For this review, use the dimensioned drawing (mm, ordinates from the lowest corner) and the shaded views. Coordinates: 2 decimals unless noted, no trailing zeros. Write each loop counter-clockwise with the first axis right and the second up, starting at its lowest first coordinate (ties: lowest second). Pieces come first, ordered by that corner, then holes.
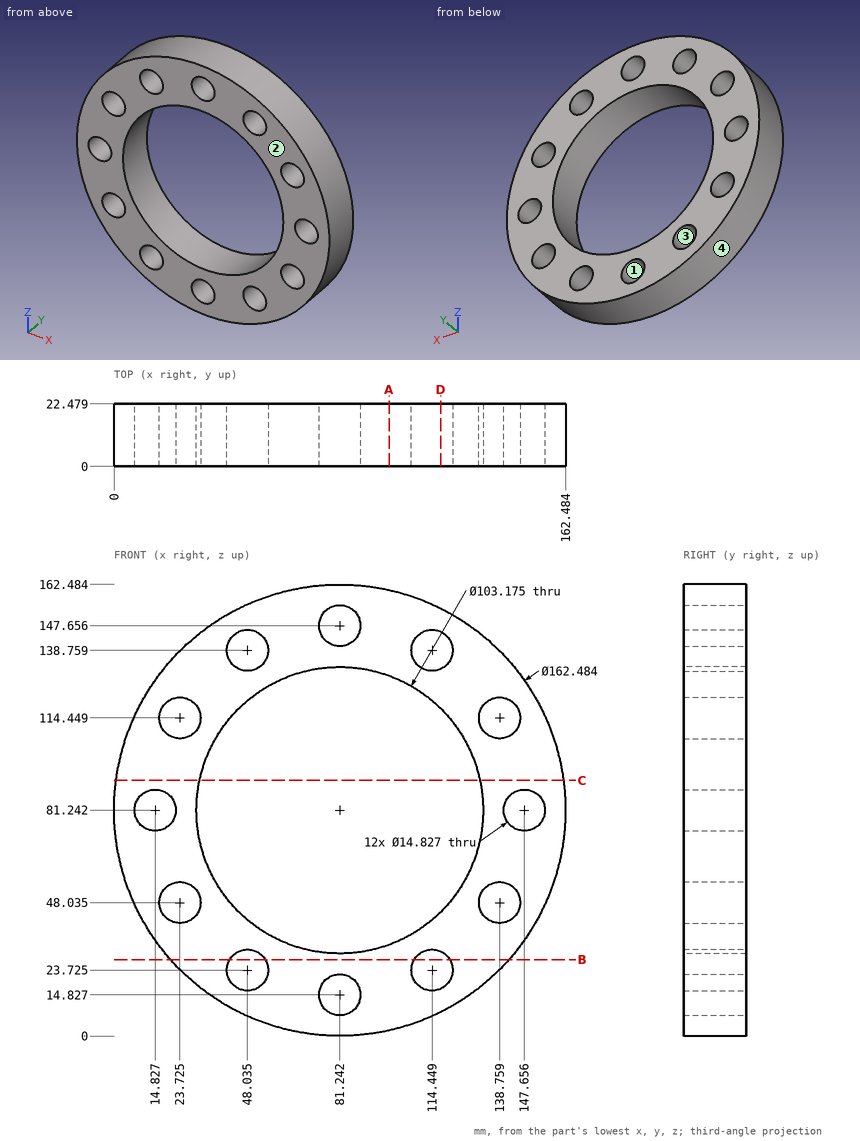
Item 1: Take a section at B-B, the plane z = 27.5. Write out the cut boundary in (x, y) (1 decimal), plus the area to 3 significant figures.
Solved:
outline: (20.3, 0) - (41.7, 0) - (41.7, 22.5) - (20.3, 22.5) - close; (54.4, 0) - (108.1, 0) - (108.1, 22.5) - (54.4, 22.5) - close; (120.8, 0) - (142.2, 0) - (142.2, 22.5) - (120.8, 22.5) - close
area: 2,170 mm2
Item 2: Take a section at A-A, the plane x = 99. Write out the cut boundary in (y, z) (1 decimal), plus the area to 3 significant figures.
Solved:
outline: (0, 2) - (22.5, 2) - (22.5, 32.8) - (0, 32.8) - close; (0, 129.7) - (22.5, 129.7) - (22.5, 160.5) - (0, 160.5) - close
area: 1,390 mm2
Item 3: Take a section at D-D, the plane x = 117.5. Write out the cut boundary in (y, z) (1 decimal), plus the area to 3 significant figures.
Solved:
outline: (0, 8.5) - (22.5, 8.5) - (22.5, 17) - (0, 17) - close; (0, 30.5) - (22.5, 30.5) - (22.5, 44.5) - (0, 44.5) - close; (0, 117.9) - (22.5, 117.9) - (22.5, 132) - (0, 132) - close; (0, 145.5) - (22.5, 145.5) - (22.5, 153.9) - (0, 153.9) - close
area: 1,010 mm2
Item 4: For pin 1 (8 mm diameter, centred on x = 27.5, z = 130.5, fed in from -Y); pin 2 (2 mm diameter, centred on x = 144.5, y = 12, fed in from -Z); pin 3 (8 mm diameter, centred on y = 12.5, z = 135.5, fed in from +X); pin 4 (1.5 mm diameter, centred on y = 7, z = 32, fed in from -X), all flat-tipped, find the tip position at first contact; note any pin that passes through.
Solved:
pin 1: stops at y = 0
pin 2: stops at z = 29.05
pin 3: stops at x = 145.07
pin 4: stops at x = 16.06
Item 5: Take a section at C-C, the plane z = 92. Write out the cut boundary in (x, y) (1 decimal).
Solved:
outline: (0.7, 0) - (30.8, 0) - (30.8, 22.5) - (0.7, 22.5) - close; (131.7, 0) - (161.8, 0) - (161.8, 22.5) - (131.7, 22.5) - close
Item 6: To check wall thickness, follow line 1 along Z through (x, y) = (48.5, 18.25) (1 decimal); line 2 along X through (y, z) = (21.5, 29) (1 decimal); line 3 along Z through (x, y) = (53, 13.25) (1 decimal). State the ranges of each line that lie inside material, in increasing order.
Solved:
line 1: z = 6.9 to 16.3, 31.1 to 41.4, 121.1 to 131.4, 146.2 to 155.6
line 2: x = 19 to 42.8, 53.2 to 109.2, 119.7 to 143.5
line 3: z = 5.1 to 18.2, 29.2 to 38.1, 124.4 to 133.3, 144.3 to 157.4
Item 7: Mouldability with a two-part tool opening along X and no side actions: class the marked faces 1, 2, 3 and 4 as pulls with the +X half, pulls with the -X half, needs draft (parallel to the pull), parting line crosses it, or undercut.
Solved:
face 1: undercut
face 2: needs draft
face 3: undercut
face 4: parting line crosses it
